The model under review builds one solid part; all positions refer to its coordinate system, in mm. A direction names the side the tool comes from. Round coordinates to 2 decimals unless told otherwise and drop trailing zeros. Loops run counter-clockwise (first coordinate to the right, second up) from the corner with the lowest first, then second, coordinate; pieces in that order, holes last. Notation, with made-up numbers: M -5.5,84.25 L -1.5,84.25 A22 cw -1.5,97.25 Z; hole C -16.75,36 d6. An arc over 180 degrees is marked long. Return JSON: item names as keys, results as strings. Group by question number.
Q1. Consider section B-B (x = -1.5). State the section outline as (y, z) points, and give its area (3 significant figures).
Q2. Clearance check with flat-ended pins moving along their axes: pin 1 Ø1.8 at (y, z) = (5, 4) entering from +X; pin 2 Ø2 at (y, z) = (44, 1.5) entering from -X; pin 3 Ø3 at (x, z) = (-7.5, 4) entering from +Y. State where each tip first meets the part, or that it passes through.
Q3. Consider section C-C (y = 9.5). State the section outline as (x, z) points.
Q4. Consider section A-A (z = 1.8). State the section outline as (x, y) points, and give its area (3 significant figures).
Q5. To check wall thickness, follow line 1 along X through (y, z) = (43, 3.25); line 2 along X through (y, z) = (27.5, 0.45); line 3 along X through (y, z) = (27, 1.9). State the ranges of each line that lie inside material, in increasing order.
Q6. Draft analysis for pull direction X (two halves, no side actions). For faces 4 (the face through (45.47, 16.91, 2.96)), 5 (the face through (0, 7, 3)), 6 (the face through (49, 0, 3)), state which applies: pulls with the +X half, pulls with the -X half, needs draft (parallel to the pull), parting line crosses it, or undercut.
Q7. For faces 1 (the face through (100, 42, 3)), 2 (the face through (-5, 35, 3)), 3 (the face through (105, 15, 3)), list the 3-axis set-ups (+Z, -Z, +X, -X, +Y, -Y) from which the entire face can be reached by the end or side of a thin tool; tool diameter is ignored.
from build123d import *

# Parameters (mm, degrees)
ESQUISSE1_W             = 10
ESQUISSE1_H             = 20
ESQUISSE1_W_2           = 100
ESQUISSE1_H_2           = 50
BOSS_EXTRU_1_DEPTH      = 6
ESQUISSE2_R             = 1.25
ENL_V_MAT_EXTRU_1_DEPTH = 6


with BuildPart() as part:
    # Esquisse1 → Boss.-Extru.1 (new body)
    with BuildSketch(Plane.XY):
        with Locations((-5, 25)):
            Rectangle(ESQUISSE1_W, ESQUISSE1_H)
        with Locations((50, 25)):
            Rectangle(ESQUISSE1_W_2, ESQUISSE1_H_2)
        with Locations((105, 25)):
            Rectangle(ESQUISSE1_W, ESQUISSE1_H)
    extrude(amount=BOSS_EXTRU_1_DEPTH)

    # Esquisse2 → Enlèv. mat.-Extru.1 (cut)
    with BuildSketch(Plane(origin=(0, 0, 0), x_dir=(-1, 0, 0), z_dir=(0, 0, -1))):
        with Locations((-44.550340057, 16.065313345)):
            Circle(ESQUISSE2_R)
        with Locations((-44.550340057, 28.065313345)):
            Circle(ESQUISSE2_R)
        with Locations((-68.550340057, 28.065313345)):
            Circle(ESQUISSE2_R)
        with Locations((-68.550340057, 16.065313345)):
            Circle(ESQUISSE2_R)
    extrude(amount=-ENL_V_MAT_EXTRU_1_DEPTH, mode=Mode.SUBTRACT)


solid = part.part
Values:
{
 "1": {"outline": "M 15,0 L 35,0 L 35,6 L 15,6 Z", "area": "120 mm2"},
 "2": {"pin 1": "stops at x = 100", "pin 2": "stops at x = 0", "pin 3": "stops at y = 35"},
 "3": {"outline": "M 0,0 L 100,0 L 100,6 L 0,6 Z"},
 "4": {"outline": "M -10,15 L 0,15 L 0,0 L 100,0 L 100,15 L 110,15 L 110,35 L 100,35 L 100,50 L 0,50 L 0,35 L -10,35 Z; hole C 44.55,16.07 d2.5; hole C 44.55,28.07 d2.5; hole C 68.55,16.07 d2.5; hole C 68.55,28.07 d2.5", "area": "5,380 mm2"},
 "5": {"line 1": "x = 0 to 100", "line 2": "x = -10 to 43.44, 45.67 to 67.44, 69.67 to 110", "line 3": "x = -10 to 43.9, 45.2 to 67.9, 69.2 to 110"},
 "6": {"face 4": "undercut", "face 5": "pulls with the -X half", "face 6": "needs draft"},
 "7": {"face 1": "+Z, -Z, +X, +Y", "face 2": "+Z, -Z, -X, +Y", "face 3": "+Z, -Z, +X, -Y"}
}
